```python
from build123d import *

# Parameters (mm, degrees)
BOSS_EXTRUDE1_DEPTH = 2.54


with BuildPart() as part:
    # Sketch1 → Boss-Extrude1 (new body)
    with BuildSketch(Plane.XY):
        with BuildLine():
            Line((0, 812.8), (0, 34.544))
            Line((0, 34.544), (15.24, 34.544))
            Line((15.24, 34.544), (15.24, 15.24))
            Line((15.24, 15.24), (34.544, 15.24))
            Line((34.544, 15.24), (34.544, 0))
            Line((34.544, 0), (587.904273944, 0))
            ThreePointArc((587.904273944, 0), (613.304273944, 25.4), (638.704273944, 0))
            Line((638.704273944, 0), (872.45698, 0))
            Line((872.45698, 0), (872.45698, 15.24))
            Line((872.45698, 15.24), (891.76098, 15.24))
            Line((891.76098, 15.24), (891.76098, 34.544))
            Line((891.76098, 34.544), (907.00098, 34.544))
            Line((907.00098, 34.544), (907.00098, 812.8))
            Line((907.00098, 812.8), (0, 812.8))
        make_face()
    extrude(amount=BOSS_EXTRUDE1_DEPTH)


solid = part.part
```
Build history of the part. All positions in model axes, mm. Give positions to 0.01 mm unless a question says otherwise; leave off trailing zeros. Write item = value, one per line. Start each with the question number.
(1) Probe L1, parallel to Y at x = 627, z = 0.7; L2, parallel to Y at x = 622, z = 0.95. List the from-to ranges inside material, lowest first. Write a range as [from, to].
(2) Pin check, flat tips, straight feed: pin 1 Ø0.8 at (y, z) = (7.5, 1) entering from -X; pin 2 Ø1.3 at (x, z) = (21.5, 1.5) entering from -Y. Stop position of each tip, or through.
(3) Two-plate mould, pull along X, no slides. Class faces 1 (the flat face through (447, 412, 0)), 2 (the cylindrical face through (612.746, 25.394, 1.252)): released by +X, released by -X, zero draft, split by the parting line, or undercut.
Responses:
q1.L1 = [21.39, 812.8]
q1.L2 = [23.87, 812.8]
q2.pin_1 = 34.54
q2.pin_2 = 15.24
q3.face_1 = zero draft
q3.face_2 = undercut
